Source: CAD feature listing. Evaluate the final solid. Frame: model axes, mm. A direction names the side the tool comes from. Round coordinates to 2 decimals unless told otherwise and drop trailing zeros. Order: outer loops, then holes, each group sorted by start corner. A loop starts at its lowest first (then second) coordinate and runs counter-clockwise, first axis right, second up. Notation, with made-up numbers: M -36,-10.75 L -19,-10.75 A14 cw -19,13.25 Z; hole C 83.5,86 d11. An arc over 180 degrees is marked long. Answer in a Markdown table with one row per item. Add a question column.
```python
from build123d import *

# Parameters (mm, degrees)
SKETCH2_W           = 166
SKETCH2_H           = 45
BOSS_EXTRUDE1_DEPTH = 35
SKETCH3_W           = 150
SKETCH3_H           = 17.75
SKETCH3_W_2         = 3.25
SKETCH3_H_2         = 5.05
BOSS_EXTRUDE4_DEPTH = 35
SKETCH8_W           = 3.1
SKETCH8_H           = 47.2
CUT_EXTRUDE2_DEPTH  = 20.15
SKETCH9_W           = 2.2
SKETCH9_H           = 14.2
SKETCH9_W_2         = 14.2
SKETCH9_H_2         = 1.1
CUT_EXTRUDE4_DEPTH  = 20.15
SKETCH11_R          = 3
SKETCH11_R_2        = 1.575
SKETCH11_R_3        = 1.65
BOSS_EXTRUDE5_DEPTH = 5
SKETCH12_R          = 3
CUT_EXTRUDE6_DEPTH  = 1
FILLET1_R           = 2.5


with BuildPart() as part:
    # Sketch2 → Boss-Extrude1 (new body)
    with BuildSketch(Plane(origin=(0, 0, 0), x_dir=(1, 0, 0), z_dir=(0, 1, 0))):
        with Locations((-83, -22.5)):
            Rectangle(SKETCH2_W, SKETCH2_H)
    extrude(amount=BOSS_EXTRUDE1_DEPTH)

    # Sketch3 → Cut-Revolve1 (revolve, cut)
    with BuildSketch(Plane(origin=(0, 35, 0), x_dir=(1, 0, 0), z_dir=(0, 1, 0))):
        with Locations((-82, -13.625)):
            Rectangle(SKETCH3_W, SKETCH3_H)
        Polygon((-7, -22.5), (-7, -4.75), (-3.25, -17.45), (-3.25, -22.5), align=None)
        with Locations((-1.625, -19.975)):
            Rectangle(SKETCH3_W_2, SKETCH3_H_2)
    revolve(axis=Axis((-166, 35, 22.5), (1, 0, 0)), mode=Mode.SUBTRACT)

    # Sketch6 → Boss-Extrude4 (add)
    with BuildSketch(Plane.XZ):
        Polygon((-150, 45), (-150, 52), (-173, 52), (-173, -7), (-150, -7), (-150, 0), (-166, 0), (-166, 45), align=None)
    extrude(amount=-BOSS_EXTRUDE4_DEPTH)

    # Sketch8 → Cut-Extrude2 (cut)
    with BuildSketch(Plane(origin=(0, 35, 0), x_dir=(1, 0, 0), z_dir=(0, 1, 0))):
        with Locations((-158.55, -22.5)):
            Rectangle(SKETCH8_W, SKETCH8_H)
    extrude(amount=-CUT_EXTRUDE2_DEPTH, mode=Mode.SUBTRACT)

    # Sketch9 → Cut-Extrude4 (cut)
    with BuildSketch(Plane.ZY.offset(173)):
        with Locations((22.5, 43.2)):
            Rectangle(SKETCH9_W, SKETCH9_H)
        with Locations((14.3, 34.45)):
            Rectangle(SKETCH9_W_2, SKETCH9_H_2)
        with Locations((22.5, 34.45)):
            Rectangle(SKETCH9_W, SKETCH9_H_2)
        with Locations((30.7, 34.45)):
            Rectangle(SKETCH9_W_2, SKETCH9_H_2)
        with Locations((30.7, 35.55)):
            Rectangle(SKETCH9_W_2, SKETCH9_H_2)
        with Locations((14.3, 35.55)):
            Rectangle(SKETCH9_W_2, SKETCH9_H_2)
        with Locations((22.5, 35.55)):
            Rectangle(SKETCH9_W, SKETCH9_H_2)
        with Locations((22.5, 26.8)):
            Rectangle(SKETCH9_W, SKETCH9_H)
    extrude(amount=-CUT_EXTRUDE4_DEPTH, mode=Mode.SUBTRACT)

    # Sketch11 → Boss-Extrude5 (add)
    # profile 1 of 21: a face of its own
    with BuildSketch(Plane(origin=(0, 0, 0), x_dir=(-1, 0, 0), z_dir=(0, -1, 0))):
        with BuildLine():
            ThreePointArc((142, -52), (142.292893219, -52.707106781), (143, -53))
            Line((143, -53), (149, -53))
            ThreePointArc((149, -53), (149.707106781, -52.707106781), (150, -52))
            Line((150, -52), (150, -45))
            Line((150, -45), (142, -45))
            Line((142, -45), (142, -47.5))
            Line((142, -47.5), (142, -52))
        make_face()
        with Locations((146, -49)):
            Circle(SKETCH11_R, mode=Mode.SUBTRACT)
    # profile 2 of 21: a face of its own
    with BuildSketch(Plane(origin=(0, 0, 0), x_dir=(-1, 0, 0), z_dir=(0, -1, 0))):
        with Locations((146, -49)):
            Circle(SKETCH11_R)
        with Locations(Location((146, -49, 0), (0, 0, 90))):
            Circle(SKETCH11_R_2, mode=Mode.SUBTRACT)
    # profile 3 of 21: a face of its own
    with BuildSketch(Plane(origin=(0, 0, 0), x_dir=(-1, 0, 0), z_dir=(0, -1, 0))):
        with BuildLine():
            ThreePointArc((139.5, -45), (141.267766953, -45.732233047), (142, -47.5))
            Line((142, -47.5), (142, -45))
            Line((142, -45), (139.5, -45))
        make_face()
    # profile 4 of 21: a face of its own
    with BuildSketch(Plane(origin=(0, 0, 0), x_dir=(-1, 0, 0), z_dir=(0, -1, 0))):
        with BuildLine():
            ThreePointArc((102.666666667, -47.5), (103.398899714, -45.732233047), (105.166666667, -45))
            Line((105.166666667, -45), (102.666666667, -45))
            Line((102.666666667, -45), (102.666666667, -47.5))
        make_face()
    # profile 5 of 21: a face of its own
    with BuildSketch(Plane(origin=(0, 0, 0), x_dir=(-1, 0, 0), z_dir=(0, -1, 0))):
        with BuildLine():
            Line((102.666666667, -47.5), (102.666666667, -45))
            Line((102.666666667, -45), (94.666666667, -45))
            Line((94.666666667, -45), (94.666666667, -47.5))
            Line((94.666666667, -47.5), (94.666666667, -49))
            ThreePointArc((94.666666667, -49), (98.666666667, -53), (102.666666667, -49))
            Line((102.666666667, -49), (102.666666667, -47.5))
        make_face()
        with Locations(Location((98.666666667, -49, 0), (0, 0, 90))):
            Circle(SKETCH11_R_2, mode=Mode.SUBTRACT)
    # profile 6 of 21: a face of its own
    with BuildSketch(Plane(origin=(0, 0, 0), x_dir=(-1, 0, 0), z_dir=(0, -1, 0))):
        with BuildLine():
            Line((94.666666667, -47.5), (94.666666667, -45))
            Line((94.666666667, -45), (92.166666667, -45))
            ThreePointArc((92.166666667, -45), (93.93443362, -45.732233047), (94.666666667, -47.5))
        make_face()
    # profile 7 of 21: a face of its own
    with BuildSketch(Plane(origin=(0, 0, 0), x_dir=(-1, 0, 0), z_dir=(0, -1, 0))):
        with BuildLine():
            ThreePointArc((55.333333333, -47.5), (56.06556638, -45.732233047), (57.833333333, -45))
            Line((57.833333333, -45), (55.333333333, -45))
            Line((55.333333333, -45), (55.333333333, -47.5))
        make_face()
    # profile 8 of 21: a face of its own
    with BuildSketch(Plane(origin=(0, 0, 0), x_dir=(-1, 0, 0), z_dir=(0, -1, 0))):
        with BuildLine():
            Line((55.333333333, -47.5), (55.333333333, -45))
            Line((55.333333333, -45), (47.333333333, -45))
            Line((47.333333333, -45), (47.333333333, -47.5))
            Line((47.333333333, -47.5), (47.333333333, -49))
            ThreePointArc((47.333333333, -49), (51.333333333, -53), (55.333333333, -49))
            Line((55.333333333, -49), (55.333333333, -47.5))
        make_face()
        with Locations(Location((51.333333333, -49, 0), (0, 0, 90))):
            Circle(SKETCH11_R_2, mode=Mode.SUBTRACT)
    # profile 9 of 21: a face of its own
    with BuildSketch(Plane(origin=(0, 0, 0), x_dir=(-1, 0, 0), z_dir=(0, -1, 0))):
        with BuildLine():
            Line((47.333333333, -47.5), (47.333333333, -45))
            Line((47.333333333, -45), (44.833333333, -45))
            ThreePointArc((44.833333333, -45), (46.601100286, -45.732233047), (47.333333333, -47.5))
        make_face()
    # profile 10 of 21: a face of its own
    with BuildSketch(Plane(origin=(0, 0, 0), x_dir=(-1, 0, 0), z_dir=(0, -1, 0))):
        with BuildLine():
            ThreePointArc((8, -47.5), (8.732233047, -45.732233047), (10.5, -45))
            Line((10.5, -45), (8, -45))
            Line((8, -45), (8, -47.5))
        make_face()
    # profile 11 of 21: a face of its own
    with BuildSketch(Plane(origin=(0, 0, 0), x_dir=(-1, 0, 0), z_dir=(0, -1, 0))):
        with BuildLine():
            Line((8, -47.5), (8, -45))
            Line((8, -45), (0, -45))
            Line((0, -45), (0, -49))
            ThreePointArc((0, -49), (4, -53), (8, -49))
            Line((8, -49), (8, -47.5))
        make_face()
        with Locations(Location((4, -49, 0), (0, 0, 90))):
            Circle(SKETCH11_R_2, mode=Mode.SUBTRACT)
    # profile 12 of 21: a face of its own
    with BuildSketch(Plane(origin=(0, 0, 0), x_dir=(-1, 0, 0), z_dir=(0, -1, 0))):
        with BuildLine():
            Line((0, 0), (8, 0))
            Line((8, 0), (8, 2.499999984))
            Line((8, 2.499999984), (8, 4))
            ThreePointArc((8, 4), (4, 8), (0, 4))
            Line((0, 4), (0, 0))
        make_face()
        with Locations(Location((4, 4, 0), (0, 0, 90))):
            Circle(SKETCH11_R_3, mode=Mode.SUBTRACT)
    # profile 13 of 21: a face of its own
    with BuildSketch(Plane(origin=(0, 0, 0), x_dir=(-1, 0, 0), z_dir=(0, -1, 0))):
        with BuildLine():
            Line((8, 0), (10.500000012, 0))
            ThreePointArc((10.500000012, 0), (8.732233057, 0.732233037), (8, 2.499999984))
            Line((8, 2.499999984), (8, 0))
        make_face()
    # profile 14 of 21: a face of its own
    with BuildSketch(Plane(origin=(0, 0, 0), x_dir=(-1, 0, 0), z_dir=(0, -1, 0))):
        with BuildLine():
            Line((44.833333315, 0), (47.333333333, 0))
            Line((47.333333333, 0), (47.333333333, 2.5))
            ThreePointArc((47.333333333, 2.5), (46.60110028, 0.732233041), (44.833333315, 0))
        make_face()
    # profile 15 of 21: a face of its own
    with BuildSketch(Plane(origin=(0, 0, 0), x_dir=(-1, 0, 0), z_dir=(0, -1, 0))):
        with BuildLine():
            Line((47.333333333, 0), (55.333333333, 0))
            Line((55.333333333, 0), (55.333333333, 2.499999938))
            Line((55.333333333, 2.499999938), (55.333333333, 4))
            ThreePointArc((55.333333333, 4), (51.333333333, 8), (47.333333333, 4))
            Line((47.333333333, 4), (47.333333333, 2.5))
            Line((47.333333333, 2.5), (47.333333333, 0))
        make_face()
        with Locations(Location((51.333333333, 4, 0), (0, 0, 90))):
            Circle(SKETCH11_R_3, mode=Mode.SUBTRACT)
    # profile 16 of 21: a face of its own
    with BuildSketch(Plane(origin=(0, 0, 0), x_dir=(-1, 0, 0), z_dir=(0, -1, 0))):
        with BuildLine():
            Line((55.333333333, 0), (57.833333333, 0))
            ThreePointArc((57.833333333, 0), (56.065566402, 0.732233025), (55.333333333, 2.499999938))
            Line((55.333333333, 2.499999938), (55.333333333, 0))
        make_face()
    # profile 17 of 21: a face of its own
    with BuildSketch(Plane(origin=(0, 0, 0), x_dir=(-1, 0, 0), z_dir=(0, -1, 0))):
        with BuildLine():
            Line((92.166666667, 0), (94.666666667, 0))
            Line((94.666666667, 0), (94.666666667, 2.5))
            ThreePointArc((94.666666667, 2.5), (93.93443362, 0.732233047), (92.166666667, 0))
        make_face()
    # profile 18 of 21: a face of its own
    with BuildSketch(Plane(origin=(0, 0, 0), x_dir=(-1, 0, 0), z_dir=(0, -1, 0))):
        with BuildLine():
            Line((94.666666667, 0), (102.666666667, 0))
            Line((102.666666667, 0), (102.666666667, 2.499999973))
            Line((102.666666667, 2.499999973), (102.666666667, 4))
            ThreePointArc((102.666666667, 4), (98.666666667, 8), (94.666666667, 4))
            Line((94.666666667, 4), (94.666666667, 2.5))
            Line((94.666666667, 2.5), (94.666666667, 0))
        make_face()
        with Locations(Location((98.666666667, 4, 0), (0, 0, 90))):
            Circle(SKETCH11_R_3, mode=Mode.SUBTRACT)
    # profile 19 of 21: a face of its own
    with BuildSketch(Plane(origin=(0, 0, 0), x_dir=(-1, 0, 0), z_dir=(0, -1, 0))):
        with BuildLine():
            Line((102.666666667, 0), (105.166666667, 0))
            ThreePointArc((105.166666667, 0), (103.398899723, 0.732233038), (102.666666667, 2.499999973))
            Line((102.666666667, 2.499999973), (102.666666667, 0))
        make_face()
    # profile 20 of 21: a face of its own
    with BuildSketch(Plane(origin=(0, 0, 0), x_dir=(-1, 0, 0), z_dir=(0, -1, 0))):
        with BuildLine():
            Line((142, 0), (150, 0))
            Line((150, 0), (150, 7))
            ThreePointArc((150, 7), (149.707106781, 7.707106781), (149, 8))
            Line((149, 8), (143, 8))
            ThreePointArc((143, 8), (142.292893219, 7.707106781), (142, 7))
            Line((142, 7), (142, 2.5))
            Line((142, 2.5), (142, 0))
        make_face()
        with Locations(Location((146, 4, 0), (0, 0, 90))):
            Circle(SKETCH11_R_3, mode=Mode.SUBTRACT)
    # profile 21 of 21: a face of its own
    with BuildSketch(Plane(origin=(0, 0, 0), x_dir=(-1, 0, 0), z_dir=(0, -1, 0))):
        with BuildLine():
            Line((139.5, 0), (142, 0))
            Line((142, 0), (142, 2.5))
            ThreePointArc((142, 2.5), (141.267766953, 0.732233047), (139.5, 0))
        make_face()
    extrude(amount=-BOSS_EXTRUDE5_DEPTH)

    # Sketch12 → Cut-Extrude6 (cut)
    with BuildSketch(Plane(origin=(0, 5, 0), x_dir=(1, 0, 0), z_dir=(0, 1, 0))):
        with Locations(Location((-146, 4, 0), (0, 0, 270))):
            Circle(SKETCH12_R)
        with Locations(Location((-98.666666667, 4, 0), (0, 0, 270))):
            Circle(SKETCH12_R)
        with Locations(Location((-51.333333333, 4, 0), (0, 0, 270))):
            Circle(SKETCH12_R)
        with Locations(Location((-4, 4, 0), (0, 0, 270))):
            Circle(SKETCH12_R)
        with Locations(Location((-4, -49, 0), (0, 0, 270))):
            Circle(SKETCH12_R)
        with Locations(Location((-51.333333333, -49, 0), (0, 0, 270))):
            Circle(SKETCH12_R)
        with Locations(Location((-98.666666667, -49, 0), (0, 0, 270))):
            Circle(SKETCH12_R)
        with Locations(Location((-146, -49, 0), (0, 0, 270))):
            Circle(SKETCH12_R)
    extrude(amount=-CUT_EXTRUDE6_DEPTH, mode=Mode.SUBTRACT)

    # Fillet1
    fillet1_edges = [part.edges().sort_by_distance(p)[0] for p in [
        (-150, 20, -7),
        (-173, 17.5, -7),
        (-173, 17.5, 52),
        (-150, 20, 52),
        (0, 20, 45),
        (0, 20, 0),
    ]]
    fillet(fillet1_edges, radius=FILLET1_R)


solid = part.part
```
(1) Pin query (flat end, axial travel): pin 1 (8 mm diameter, centred on x = -50.5, z = 11.5, fed in from +Y); pin 2 (5 mm diameter, centred on y = 16, z = 46.5, fed in from +X); pin 3 (6 mm diameter, centred on x = -74.5, z = 5.5, fed in from -Y); pin 4 (3 mm diameter, centred on x = -39.5, z = 31, fed in from +Y) (3 decimals). Return the tip coordinate at first contact, or that it passes through.
(2) Cut plane A-A (x = -146). Return loops of the section in (y, z) (3 decimals), and give its area (3 significant figures).
(3) Line query: line 1 (X direction, y = 19.5, z = -1); line 2 (Z direction, x = -153.5, y = 8); line 3 (X direction, y = 20.5, z = 40). Output: solid intervals per line, ascending. Write a range as from..to.
(4) Access query for faces 1 (the face through (-150, 20, 47)), 2 (the face through (-4.1, 5, -0.8)), 3 (the face through (-160, 17, 52)), 4 (the face through (-1.6, 29.95, 22.61)), 5 (the face through (-100, 4, -2.7)). Directions: +Z, -Z, +X, -X, +Y, -Y. A direction counts if a zero-diameter tool reaches every point of the face in a straight line with its end or side. Return the directions, or none.
(5) Cut plane C-C (x = -24). Return loops of the section in (y, z), and give its area (3 significant figures).
(6) Draft query along Z for faces 6 (the face through (-146, 2, 53)), 7 (the face through (-77, 17, 0)), 8 (the face through (-3.931, 1.972, 50.573)), 9 (the face through (-80.95, 17.254, 22.89)). Return one class per face: +Z half, -Z half, draft (parallel to the pull), parting line (faces both ways), or undercut.
(7) Cut plane B-B (y = 11.5). Return loops of the section in (x, z), and give its area (3 significant figures).
Answer list:
| question | item | result |
|---|---|---|
| 1 | pin 1 | y = 25.51 |
| 1 | pin 2 | x = -0.5 |
| 1 | pin 3 | y = 0 |
| 1 | pin 4 | y = 20.335 |
| 2 | outline | M 0,-8 L 5,-8 L 5,-7 L 4,-7 L 4,-5.65 L 0,-5.65 Z; M 0,-2.35 L 4,-2.35 L 4,-1 L 5,-1 L 5,0 L 35,0 L 35,4.75 A17.75 cw 35,40.25 L 35,45 L 5,45 L 5,46 L 4,46 L 4,47.425 L 0,47.425 Z; M 0,50.575 L 4,50.575 L 4,52 L 5,52 L 5,53 L 0,53 Z |
| 2 | area | 1,120 mm² |
| 3 | line 1 | -173..-160.1, -157..-150 |
| 3 | line 2 | -7..52 |
| 3 | line 3 | -173..-160.1, -157..0 |
| 4 | face 1 | +Z, +X, +Y |
| 4 | face 2 | -Z, +X, +Y |
| 4 | face 3 | +Z, -X, +Y, -Y |
| 4 | face 4 | +X, +Y |
| 4 | face 5 | +Y |
| 5 | outline | M 0,0 L 35,0 L 35,4.75 A17.75 cw 35,40.25 L 35,45 L 0,45 Z |
| 5 | area | 1,080 mm² |
| 6 | face 6 | +Z half |
| 6 | face 7 | -Z half |
| 6 | face 8 | undercut |
| 6 | face 9 | undercut |
| 7 | outline | M -173,-4.5 A2.5 ccw -170.5,-7 L -152.5,-7 A2.5 ccw -150,-4.5 L -150,0 L -2.5,0 A2.5 ccw 0,2.5 L 0,42.5 A2.5 ccw -2.5,45 L -150,45 L -150,49.5 A2.5 ccw -152.5,52 L -170.5,52 A2.5 ccw -173,49.5 Z |
| 7 | area | 8,100 mm² |
